Check sheet for the modelled part. Datum: model origin and axes. Units: mm. A direction names the side the tool comes from. Give positions to 0.01 mm unless a question says otherwise; leave off trailing zeros. Loops run counter-clockwise (first coordinate to the right, second up) from the corner with the lowest first, then second, coordinate; pieces in that order, holes last. Notation, with made-up numbers: (-20, 8) -> (-1, 8) arc R27 cw to (-1, 36) -> close; hole circle Ø8 at (13.5, 61). An arc over 180 degrees is marked (long way). Answer as CSV lines item,"result". Start each with the question number.
(1) Section check D-D on z = -12. Enter the section's corners in (x, y), plus the area to 3 significant figures.
(2) Section check C-C on y = 9. Enter the section's corners in (x, z), plus the area to 3 significant figures.
(3) Access from +Z, -Z, +X, -X, +Y, -Y to the whole of each face (thin tool, end or side, straight path). Record for faces 5 (the face through (20.956, 20.036, -6.599)), 6 (the face through (13.621, 26.328, -21.364)).
(4) Gauge pin test, flat ends, axial feed: pin 1 Ø8 at (x, y) = (-16.5, 11) entering from +Z; pin 2 Ø3 at (x, y) = (-13, 7.5) entering from +Z; pin 3 Ø15 at (x, z) = (10, 7) entering from -Y. Record the tip position at first contact, or that the pin passes through.
(5) Section check A-A on x = 0. Enter the section's corners in (y, z).
(6) Release check for a two-part mould opening along X. For faces 1 (the face through (9, 40.64, 0)), 2 (the face through (-19.451, 2.504, 14.915)), 3 (the face through (-1.72, 43.86, 7.75)), 4 (the face through (-13, 5.08, -21)) record: pulls with the +X half, pulls with the -X half, needs draft (parallel to the pull), parting line crosses it, or undercut.
(7) Section check B-B on z = 0. Enter the section's corners in (x, y).
(8) Material ranges on line 1 (Z direction, x = 0, y = 13); line 2 (Z direction, x = 0, y = 42.25), recorded low to high. Write a range as from..to.
from build123d import *

# Parameters (mm, degrees)
SKETCH1_R           = 24.511
SKETCH1_R_2         = 21.971
BOSS_EXTRUDE1_DEPTH = 40.64
SKETCH2_R           = 24.511
BOSS_EXTRUDE2_DEPTH = 6.35
CUT_EXTRUDE1_REACH  = 48.99
SKETCH3_R           = 7.9375
SKETCH4_R           = 25.3365
SKETCH4_R_2         = 24.511
BOSS_EXTRUDE3_DEPTH = 41.91


with BuildPart() as part:
    # Sketch1 → Boss-Extrude1 (new body)
    with BuildSketch(Plane(origin=(0, 0, 0), x_dir=(1, 0, 0), z_dir=(0, 1, 0))):
        Circle(SKETCH1_R)
        Circle(SKETCH1_R_2, mode=Mode.SUBTRACT)
    extrude(amount=BOSS_EXTRUDE1_DEPTH)

    # Sketch2 → Boss-Extrude2 (add)
    with BuildSketch(Plane(origin=(0, 40.64, 0), x_dir=(1, 0, 0), z_dir=(0, 1, 0))):
        Circle(SKETCH2_R)
    extrude(amount=BOSS_EXTRUDE2_DEPTH)

    # Sketch3 → Cut-Extrude1 (cut, up to next)
    with BuildSketch(Plane(origin=(0, 46.99, 0), x_dir=(1, 0, 0), z_dir=(0, 1, 0)), mode=Mode.PRIVATE) as cut_extrude1_sk1:
        Circle(SKETCH3_R)
    cut_extrude1_tool1 = extrude(cut_extrude1_sk1.sketch, amount=-CUT_EXTRUDE1_REACH, mode=Mode.PRIVATE) & part.part
    add(cut_extrude1_tool1.solids().sort_by_distance((0, 46.99, 0))[0], mode=Mode.SUBTRACT)

    # Sketch4 → Boss-Extrude3 (add)
    with BuildSketch(Plane(origin=(0, 46.99, 0), x_dir=(1, 0, 0), z_dir=(0, 1, 0))):
        Circle(SKETCH4_R)
        Circle(SKETCH4_R_2, mode=Mode.SUBTRACT)
    extrude(amount=-BOSS_EXTRUDE3_DEPTH)


solid = part.part
Working result:
1,outline,"(-22.31, 5.08) -> (-21.37, 5.08) -> (-21.37, 0) -> (-18.4, 0) -> (-18.4, 40.64) -> (18.4, 40.64) -> (18.4, 0) -> (21.37, 0) -> (21.37, 5.08) -> (22.31, 5.08) -> (22.31, 46.99) -> (-22.31, 46.99) -> close"
1,area,"592 mm^2"
2,outline,"circle Ø50.67 at (0, 0); hole circle Ø43.94 at (0, 0)"
2,area,"500 mm^2"
3,face 5,"-Y"
3,face 6,"+Y, -Y"
4,pin 1,"stops at z = 22.04"
4,pin 2,"stops at z = 22.58"
4,pin 3,"stops at y = 40.64"
5,outline,"(0, -24.51) -> (5.08, -24.51) -> (5.08, -25.34) -> (46.99, -25.34) -> (46.99, -7.94) -> (40.64, -7.94) -> (40.64, -21.97) -> (0, -21.97) -> close; (0, 21.97) -> (40.64, 21.97) -> (40.64, 7.94) -> (46.99, 7.94) -> (46.99, 25.34) -> (5.08, 25.34) -> (5.08, 24.51) -> (0, 24.51) -> close"
6,face 1,"undercut"
6,face 2,"parting line crosses it"
6,face 3,"undercut"
6,face 4,"needs draft"
7,outline,"(-25.34, 5.08) -> (-24.51, 5.08) -> (-24.51, 0) -> (-21.97, 0) -> (-21.97, 40.64) -> (-7.94, 40.64) -> (-7.94, 46.99) -> (-25.34, 46.99) -> close; (7.94, 40.64) -> (21.97, 40.64) -> (21.97, 0) -> (24.51, 0) -> (24.51, 5.08) -> (25.34, 5.08) -> (25.34, 46.99) -> (7.94, 46.99) -> close"
8,line 1,"z = -25.34..-21.97, 21.97..25.34"
8,line 2,"z = -25.34..-7.94, 7.94..25.34"
